Geometry: final body of the model. Coordinates: model frame, mm. Face numbers are marked on the shaded views. A direction names the side the tool comes from. Give positions to 0.01 mm unless a question says otherwise; leave off trailing zeros. Write each loop counter-clockwise with the first axis right and the second up, starting at its lowest first coordinate (ties: lowest second). Pieces come first, ordered by that corner, then holes.
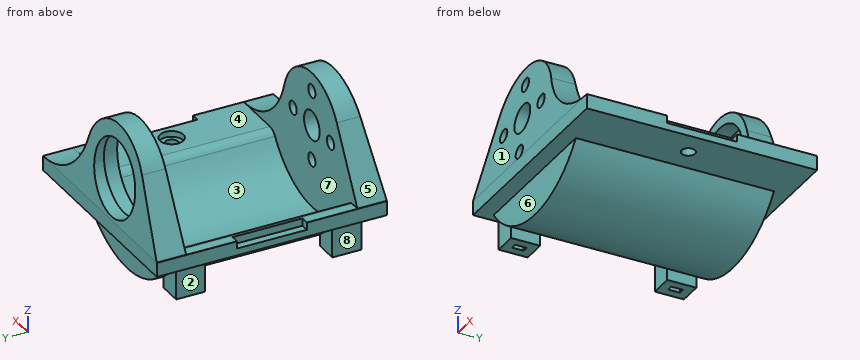
from build123d import *

# Parameters (mm, degrees)
SKETCH_1_R               = 16.3
EXTRUDE_1_DEPTH          = 19.75
SKETCH_2_W               = 36.5
SKETCH_2_H               = 2.5
EXTRUDE_2_DEPTH          = 39.5
SKETCH_3_W               = 44.844436064
SKETCH_3_H               = 25.506740045
CUT_EXTRUDE_1_DEPTH      = 50
EXTRUDE_3_DEPTH          = 5.05
SKETCH_5_R               = 14.25
CUT_EXTRUDE_2_DEPTH      = 29.4
SKETCH_6_R               = 2.5
CUT_EXTRUDE_3_DEPTH      = 44.930797853
CUT_EXTRUDE_6_REACH      = 49.993
SKETCH_9_R               = 7.5
SKETCH_12_R              = 1.15
CUT_EXTRUDE_9_DEPTH      = 34.662664779
SKETCH_13_R              = 2
CUT_EXTRUDE_10_DEPTH     = 1
SKETCH_14_W              = 2.8
SKETCH_14_H              = 12
CUT_EXTRUDE_11_DEPTH     = 1.3
SKETCH_15_W              = 2.8
SKETCH_15_H              = 12
CUT_EXTRUDE_12_DEPTH     = 1.3
EXTRUDE_5_REACH          = 40.183
EXTRUDE_5_END_RADIUS     = 16.3
SKETCH_16_W              = 4
SKETCH_16_H              = 5
SKETCH_17_W              = 1
SKETCH_17_H              = 2
CUT_EXTRUDE_13_DEPTH     = 2.5
SKETCH_19_R              = 8.51898124
SKETCH_19_R_2            = 6.5
EXTRUDE_6_DEPTH          = 2.25
CUT_EXTRUDE_18_REACH     = 49.993
SKETCH_20_R              = 1.15
PATTERN_CIRCULAR_1_COUNT = 4
CUT_EXTRUDE_8_DEPTH      = 45.587021654
SKETCH_18_W              = 26.346157216
SKETCH_18_H              = 2.75
CUT_EXTRUDE_16_DEPTH     = 12.5
FILLET_1_R               = 2
FILLET_2_R               = 1


with BuildPart() as part:
    # 草图1 → 凸台-拉伸1 (new, symmetric)
    with BuildSketch(Plane(origin=(0, 0, 0), x_dir=(1, 0, 0), z_dir=(0, 1, 0))):
        with Locations(Location((0, 0, 0), (0, 0, 270))):
            Circle(SKETCH_1_R)
    extrude(amount=EXTRUDE_1_DEPTH, both=True)

    # 草图2 → 凸台-拉伸2 (add, through all)
    with BuildSketch(Plane.XZ.offset(19.75)):
        with Locations((3.6, -8.35)):
            Rectangle(SKETCH_2_W, SKETCH_2_H)
    extrude(amount=-EXTRUDE_2_DEPTH)

    # 草图3 → 切除-拉伸1 (cut)
    with BuildSketch(Plane.XZ.offset(19.75)):
        with Locations((-0.572218032, 5.653370022)):
            Rectangle(SKETCH_3_W, SKETCH_3_H)
    extrude(amount=-CUT_EXTRUDE_1_DEPTH, mode=Mode.SUBTRACT)

    # 草图4 → 凸台-拉伸3 (add)
    with BuildSketch(Plane.XZ.offset(19.75)):
        with BuildLine():
            Line((-14.65, -7.146152811), (-7.996542478, 4.549209646))
            ThreePointArc((-7.996542478, 4.549209646), (1.047927533, 9.140122969), (8.818653972, 2.621324497))
            ThreePointArc((8.818653972, 2.621324497), (13.721037439, -4.401937543), (21.85, -7.1))
            Line((21.85, -7.1), (-14.65, -7.146152811))
        make_face()
    extrude_3 = extrude(amount=-EXTRUDE_3_DEPTH)

    # 镜向1: 凸台-拉伸3 across plane
    add(extrude_3.mirror(Plane.ZX))

    # 草图5 → 切除-拉伸2 (cut)
    with BuildSketch(Plane(origin=(0, -14.7, 0), x_dir=(1, 0, 0), z_dir=(0, 1, 0))):
        Circle(SKETCH_5_R)
    extrude(amount=CUT_EXTRUDE_2_DEPTH, mode=Mode.SUBTRACT)

    # 草图6 → 切除-拉伸3 (cut, through all)
    with BuildSketch(Plane(origin=(0, -14.7, 0), x_dir=(1, 0, 0), z_dir=(0, 1, 0))):
        with Locations(Location((0, 0, 0), (0, 0, 270))):
            Circle(SKETCH_6_R)
    extrude(amount=-CUT_EXTRUDE_3_DEPTH, mode=Mode.SUBTRACT)

    # 草图9 → 切除-拉伸6 (cut, up to next)
    with BuildSketch(Plane(origin=(0, 19.75, 0), x_dir=(1, 0, 0), z_dir=(0, 1, 0)), mode=Mode.PRIVATE) as cut_extrude_6_sk1:
        with Locations(Location((0, 0, 0), (0, 0, 270))):
            Circle(SKETCH_9_R)
    cut_extrude_6_tool1 = extrude(cut_extrude_6_sk1.sketch, amount=-CUT_EXTRUDE_6_REACH, mode=Mode.PRIVATE) & part.part
    add(cut_extrude_6_tool1.solids().sort_by_distance((0, 19.75, 0))[0], mode=Mode.SUBTRACT)

    # 草图12 → 切除-拉伸9 (cut, through all)
    with BuildSketch(Plane.XY.offset(-7.1)):
        with Locations((17.5, 0)):
            Circle(SKETCH_12_R)
    extrude(amount=-CUT_EXTRUDE_9_DEPTH, mode=Mode.SUBTRACT)

    # 草图13 → 切除-拉伸10 (cut)
    with BuildSketch(Plane.XY.offset(-7.1)):
        with Locations((17.5, 0)):
            Circle(SKETCH_13_R)
    extrude(amount=-CUT_EXTRUDE_10_DEPTH, mode=Mode.SUBTRACT)

    # 草图14 → 切除-拉伸11 (cut)
    with BuildSketch(Plane.XY.offset(-7.1)):
        with Locations((21.85, 0)):
            Rectangle(SKETCH_14_W, SKETCH_14_H)
    extrude(amount=-CUT_EXTRUDE_11_DEPTH, mode=Mode.SUBTRACT)

    # 草图15 → 切除-拉伸12 (cut)
    with BuildSketch(Plane.XY.offset(-7.1)):
        with Locations((-14.672423113, 0)):
            Rectangle(SKETCH_15_W, SKETCH_15_H)
    extrude(amount=-CUT_EXTRUDE_12_DEPTH, mode=Mode.SUBTRACT)

    # 凸台-拉伸5: up to this cylinder (the profile starts outside it)
    extrude_5_end = Plane(origin=(0, 13.4, 0), z_dir=(0, -1, 0)) * Cylinder(EXTRUDE_5_END_RADIUS, 113.966, mode=Mode.PRIVATE)
    # 草图16 → 凸台-拉伸5 (add, up to the surface)
    with BuildSketch(Plane(origin=(0, 0, -15.1), x_dir=(-1, 0, 0), z_dir=(0, 0, -1)), mode=Mode.PRIVATE) as extrude_5_sk1:
        with Locations((11.65, 13.4)):
            Rectangle(SKETCH_16_W, SKETCH_16_H)
    extrude_5_tool1 = extrude(extrude_5_sk1.sketch, amount=-EXTRUDE_5_REACH, mode=Mode.PRIVATE) - extrude_5_end
    extrude_5 = extrude_5_tool1.solids().sort_by_distance((-11.65, 13.4, -15.1))[0]
    add(extrude_5)

    # 镜向4: 凸台-拉伸5 across plane
    add(extrude_5.mirror(Plane.ZX))

    # 草图17 → 切除-拉伸13 (cut)
    with BuildSketch(Plane(origin=(0, 0, -15.1), x_dir=(-1, 0, 0), z_dir=(0, 0, -1))):
        with Locations((11.65, 13.4)):
            Rectangle(SKETCH_17_W, SKETCH_17_H)
    cut_extrude_13 = extrude(amount=-CUT_EXTRUDE_13_DEPTH, mode=Mode.SUBTRACT)

    # 镜向5: 切除-拉伸13 across plane
    add(cut_extrude_13.mirror(Plane.ZX), mode=Mode.SUBTRACT)

    # 草图19 → 凸台-拉伸6 (add)
    with BuildSketch(Plane(origin=(0, 19.75, 0), x_dir=(1, 0, 0), z_dir=(0, 1, 0))):
        Circle(SKETCH_19_R)
        with Locations(Location((0, 0, 0), (0, 0, 270))):
            Circle(SKETCH_19_R_2, mode=Mode.SUBTRACT)
    extrude(amount=-EXTRUDE_6_DEPTH)

    # 草图20 → 切除-拉伸18 (cut, up to next)
    with BuildSketch(Plane.XZ.offset(19.75), mode=Mode.PRIVATE) as cut_extrude_18_sk1:
        with Locations(Location((0, 6, 0), (0, 0, 270))):
            Circle(SKETCH_20_R)
    cut_extrude_18_tool1 = extrude(cut_extrude_18_sk1.sketch, amount=-CUT_EXTRUDE_18_REACH, mode=Mode.PRIVATE) & part.part
    cut_extrude_18 = cut_extrude_18_tool1.solids().sort_by_distance((0, -19.75, 6))[0]
    add(cut_extrude_18, mode=Mode.SUBTRACT)

    # 阵列(圆周)1: 切除-拉伸18 ×4 about axis
    pattern_circular_1_axis = Axis((0, 0, 0), (0, 1, 0))
    for i in range(1, PATTERN_CIRCULAR_1_COUNT):
        add(cut_extrude_18.rotate(pattern_circular_1_axis, i * 360 / PATTERN_CIRCULAR_1_COUNT), mode=Mode.SUBTRACT)

    # 草图7 → 切除-拉伸8 (cut, through all)
    with BuildSketch(Plane.ZY.offset(14.65)):
        Polygon((-7.1, 19.75), (9.2, 18.323934785), (9.2, 19.75), align=None)
    cut_extrude_8 = extrude(amount=-CUT_EXTRUDE_8_DEPTH, mode=Mode.SUBTRACT)

    # 镜向3: 切除-拉伸8 across plane
    add(cut_extrude_8.mirror(Plane.ZX), mode=Mode.SUBTRACT)

    # 草图18 → 切除-拉伸16 (cut)
    with BuildSketch(Plane(origin=(0, 0, -9.6), x_dir=(-1, 0, 0), z_dir=(0, 0, -1))):
        with Locations((0, 18.375)):
            Rectangle(SKETCH_18_W, SKETCH_18_H)
    cut_extrude_16 = extrude(amount=CUT_EXTRUDE_16_DEPTH, mode=Mode.SUBTRACT)

    # 镜向6: 切除-拉伸16 across plane
    add(cut_extrude_16.mirror(Plane.ZX), mode=Mode.SUBTRACT)

    # 圆角1
    fillet_1_edges = [part.edges().sort_by_distance(p)[0] for p in [
        (12.355262037, 0, -7.1),
    ]]
    fillet(fillet_1_edges, radius=FILLET_1_R)

    # 圆角2
    fillet_2_edges = [part.edges().sort_by_distance(p)[0] for p in [
        (-12.355262037, 0, -7.1),
    ]]
    fillet(fillet_2_edges, radius=FILLET_2_R)


solid = part.part
Q1. Ray query, line 1 along Y through (x, z) = (17.5, -8.6); line 2 along Y through (x, z) = (17.5, -7.9); line 3 along Z through (x, y) = (19.5, 8). Return the intervals inside material, ascending.
Filled sheet:
line 1: y = -19.75 to -1.15, 1.15 to 19.75
line 2: y = -19.75 to -2, 2 to 19.75
line 3: z = -9.6 to -7.1
Q2. Section D-D on x = 17.5. Output: boundary loops of the cut face in (y, z), plus the area to 3 significant figures.
Filled sheet:
outline: (-19.75, -9.6) - (-1.15, -9.6) - (-1.15, -8.1) - (-2, -8.1) - (-2, -7.1) - (-14.7, -7.1) - (-14.7, -6.39) - (-19.69, -6.39) - (-19.75, -7.1) - close; (1.15, -9.6) - (19.75, -9.6) - (19.75, -7.1) - (19.69, -6.39) - (14.7, -6.39) - (14.7, -7.1) - (2, -7.1) - (2, -8.1) - (1.15, -8.1) - close
area: 98.5 mm2
Q3. Pin query (flat end, axial travel): P1, Ø0.8, axis at x = -12, y = 13.5, coming from the -Z side; P2, Ø8, axis at x = 4.5, y = 3.5, coming from the +Z side; P3, Ø1, axis at y = -4.5, z = -13, coming from the +X side. Return the tip coordinate at first contact, or that it passes through.
Filled sheet:
P1: stops at z = -15.1
P2: stops at z = -11.44
P3: stops at x = 10.46
Q4. Section C-C on z = 0. Output: boundary loops of the cut face in (x, y), plus the area to 3 significant figures.
Filled sheet:
outline: (-10.58, -19.13) - (-7.15, -19.13) - (-7.15, -14.7) - (-10.58, -14.7) - close; (-10.58, 14.7) - (-7.5, 14.7) - (-7.5, 17.5) - (-6.5, 17.5) - (-6.5, 19.13) - (-10.58, 19.13) - close; (-4.85, -19.13) - (-2.5, -19.13) - (-2.5, -14.7) - (-4.85, -14.7) - close; (2.5, -19.13) - (4.85, -19.13) - (4.85, -14.7) - (2.5, -14.7) - close; (6.5, 17.5) - (7.5, 17.5) - (7.5, 14.7) - (9.91, 14.7) - (9.91, 19.13) - (6.5, 19.13) - close; (7.15, -19.13) - (9.91, -19.13) - (9.91, -14.7) - (7.15, -14.7) - close
area: 75.8 mm2
Q5. Access query for the marked faces 4, 5, 6, 7 and 8. Directions: +Z, -Z, +X, -X, +Y, -Y. A direction counts if a zero-diameter tool reaches every point of the face in a straight line with its end or side. Return the directions, or none.
Filled sheet:
face 4: +Z, +X, -X
face 5: +Z, -X, +Y, -Y
face 6: -Z, +X, -X, -Y
face 7: +Z
face 8: -Z, -X, +Y, -Y
Q6. Section B-B on z = -10.5. Output: boundary loops of the cut face in (x, y), plus the area to 3 significant figures.
Filled sheet:
outline: (-13.65, -15.9) - (-12.47, -15.9) - (-12.47, -17) - (12.47, -17) - (12.47, 17) - (-12.47, 17) - (-12.47, 15.9) - (-13.65, 15.9) - (-13.65, 10.9) - (-12.47, 10.9) - (-12.47, -10.9) - (-13.65, -10.9) - close; hole (-9.63, -14.7) - (9.63, -14.7) - (9.63, 14.7) - (-9.63, 14.7) - close
area: 293 mm2
Q7. Pull-direction query (Y, two-part tool) for the marked faces 1, 2 and 3; classes: released by +Y, released by -Y, zero draft, split by the parting line, or undercut.
Filled sheet:
face 1: released by -Y
face 2: zero draft
face 3: undercut
Q8. Section A-A on y = 3.5. Output: boundary loops of the cut face in (x, z).
Filled sheet:
outline: (-14.65, -9.6) - (-13.17, -9.6) arc R16.3 ccw to (13.17, -9.6) - (21.85, -9.6) - (21.85, -8.4) - (20.45, -8.4) - (20.45, -7.1) - (13.46, -7.1) arc R2 ccw to (11.81, -7.98) arc R14.25 cw to (-12.07, -7.57) arc R1 ccw to (-12.92, -7.1) - (-13.27, -7.1) - (-13.27, -8.4) - (-14.65, -8.4) - close
